For this review, take the finished solid that the model builds, in its own axes (mm). A direction names the side the tool comes from. Give positions to 0.01 mm unless a question says otherwise; leave off trailing zeros. Write each loop counter-clockwise with the first axis right and the second up, starting at its lowest first coordinate (ties: lowest second). Pieces come first, ordered by that corner, then holes.
1) Machinability: for faces 1 (the face through (14, 3.175, 150)), 2 (the face through (7, 2, 0)), which of the approach directions +Z, -Z, +X, -X, +Y, -Y give a long, thin tool a straight path to every point of the face, cutting with its end or side? Answer none if there is none.
2) Wall thickness on line 1 along X through (y, z) = (1.2, 25.4); line 2 along Y through (x, z) = (2.15, 279.4); line 3 along X through (y, z) = (12, 276) (3 decimals): over which ranges is each line inside the solid? List them lowest first.
3) We need section A-A on z = 94. Give the boundary of the cut face in (x, y) (3 decimals), and give its area (3 significant figures).
4) For P1, Ø4, axis at x = 15, z = 261.5, coming from the +Y side (3 decimals); P2, Ø5, axis at y = 12.7, z = 279.4, coming from the +X side (3 decimals), all flat-tipped, find the tip position at first contact; note any pin that passes through.
5) We need section B-B on y = 17.5. Give the boundary of the cut face in (x, z) (3 decimals).
Autodesk Inventor part; units mm, degrees
ref_plane "YZ Plane" through (0, 0, 0) normal (1, 0, 0) x (0, 1, 0)
ref_plane "XZ Plane" through (0, 0, 0) normal (0, 1, 0) x (-1, 0, 0)
ref_plane "XY Plane" through (0, 0, 0) normal (0, 0, 1) x (1, 0, 0)
sketch "Sketch1" plane through (0, 0, 0) normal (0, 0, 1) x (1, 0, 0)
  line L0 (0, 25.4) -> (0, 0)
  line L1 (0, 0) -> (25.4, 0)
  line L2 (25.4, 0) -> (25.4, 3.175)
  line L3 (25.4, 3.175) -> (3.175, 3.175)
  line L4 (3.175, 3.175) -> (3.175, 25.4)
  line L5 (3.175, 25.4) -> (0, 25.4)
  dimension "d11" = 25.4
  dimension "d12" = 25.4
  dimension "d13" = 3.175
  dimension "d14" = 3.175
extrude "Extrusion1" add sketch "Sketch1" along normal blind 304.8
hole "Hole1" at (6.35, 0, 25.4) direction (0, 1, 0) diameter 3.175 end through all
hole "Hole2" at (0, 12.7, 25.4) direction (1, 0, 0) diameter 3.175 end through all
pattern_linear "Rectangular Pattern1" count 11 spacing 25.4 along (0, 0, 1) of "Hole1"
pattern_linear "Rectangular Pattern2" count 11 spacing 25.4 along (0, 0, 1) of "Hole2"
properties part number "Fer Angle"
Results list:
1. face 1: +Z, -Z, +X, +Y
1. face 2: -Z, +X, -X, +Y, -Y
2. line 1: x = 0 to 4.76, 7.94 to 25.4
2. line 2: y = 0 to 11.11, 14.29 to 25.4
2. line 3: x = 0 to 3.175
3. outline: (0, 0) - (25.4, 0) - (25.4, 3.175) - (3.175, 3.175) - (3.175, 25.4) - (0, 25.4) - close
3. area: 151 mm2
4. P1: stops at y = 3.175
4. P2: stops at x = 3.175
5. outline: (0, 0) - (3.175, 0) - (3.175, 304.8) - (0, 304.8) - close
